The model under review builds one solid part; all positions refer to its coordinate system, in mm. Face numbers are marked on the shaded views. A direction names the side the tool comes from. Coordinates: 2 decimals unless noted, no trailing zeros. Order: outer loops, then holes, each group sorted by start corner. A loop starts at its lowest first (then second) coordinate and runs counter-clockwise, first axis right, second up. Notation, with made-up numbers: (39.5, 61) -> (86.5, 61) arc R28 cw to (86.5, 88) -> close; hole circle Ø8 at (54, 4). An arc over 180 degrees is marked (long way). Use one line per item in the form item = value.
from build123d import *

# Parameters (mm, degrees)
SKETCH1_R           = 12.7
BOSS_EXTRUDE1_DEPTH = 5
SKETCH1_3_R         = 6
CUT_EXTRUDE1_DEPTH  = 5
SKETCH1_4_R         = 7.5
SKETCH1_4_R_2       = 6
CUT_EXTRUDE2_DEPTH  = 2.5
CHAMFER1_SIZE       = 0.25


with BuildPart() as part:
    # Sketch1 → Boss-Extrude1 (new body)
    with BuildSketch(Plane(origin=(0, 0, 0), x_dir=(1, 0, 0), z_dir=(0, 1, 0))):
        with Locations(Location((0, 0, 0), (0, 0, 270))):
            Circle(SKETCH1_R)
    extrude(amount=BOSS_EXTRUDE1_DEPTH)

    # Sketch1<3> → Cut-Extrude1 (cut)
    with BuildSketch(Plane(origin=(0, 0, 0), x_dir=(1, 0, 0), z_dir=(0, 1, 0))):
        with Locations(Location((0, 0, 0), (0, 0, 270))):
            Circle(SKETCH1_3_R)
    extrude(amount=CUT_EXTRUDE1_DEPTH, mode=Mode.SUBTRACT)

    # Sketch1<4> → Cut-Extrude2 (cut)
    with BuildSketch(Plane(origin=(0, 0, 0), x_dir=(1, 0, 0), z_dir=(0, 1, 0))):
        with Locations(Location((0, 0, 0), (0, 0, 270))):
            Circle(SKETCH1_4_R)
        with Locations(Location((0, 0, 0), (0, 0, 270))):
            Circle(SKETCH1_4_R_2, mode=Mode.SUBTRACT)
    extrude(amount=CUT_EXTRUDE2_DEPTH, mode=Mode.SUBTRACT)

    # Chamfer1
    chamfer1_edges = [part.edges().sort_by_distance(p)[0] for p in [
        (0, 0, -7.5),
        (0, 0, -12.7),
        (0, 5, -12.7),
    ]]
    chamfer(chamfer1_edges, length=CHAMFER1_SIZE)


solid = part.part
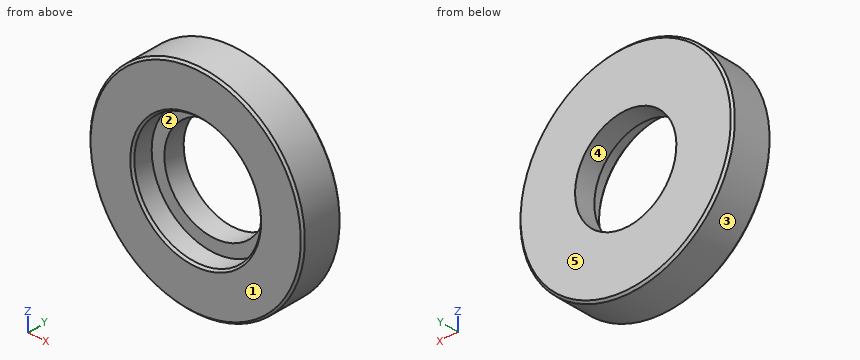
Item 1: We need section C-C (y = 4.35). Write out the cut boundary in (x, z), plus the area to 3 significant figures.
Results found:
outline = circle Ø25.4 at (0, 0); hole circle Ø12 at (0, 0)
area = 394 mm²
Item 2: To check wall thickness, follow L1, parallel to X at y = 1.35, z = 0; L2, parallel to X at y = 4.25, z = 0; L3, parallel to Y at x = -3.5, z = -6.5. State the ranges of each line that lie inside material, in increasing order. Write a range as from..to.
Results found:
L1 = -12.7..-7.5, 7.5..12.7
L2 = -12.7..-6, 6..12.7
L3 = 2.5..5
Item 3: Tool access review of the marked faces 1 and 2: name each direction out of +Z, -Z, +X, -X, +Y, -Y from which nothing blocks a thin tool from reaching the whole face with its end or side.
Results found:
face_1 = +Z, -Z, +X, -X, -Y
face_2 = -Y
Item 4: We need section B-B (x = 0). Write out the cut boundary in (y, z), plus the area to 3 significant figures.
Results found:
outline = (0, -12.45) -> (0.25, -12.7) -> (4.75, -12.7) -> (5, -12.45) -> (5, -6) -> (2.5, -6) -> (2.5, -7.5) -> (0.25, -7.5) -> (0, -7.75) -> close; (0, 7.75) -> (0.25, 7.5) -> (2.5, 7.5) -> (2.5, 6) -> (5, 6) -> (5, 12.45) -> (4.75, 12.7) -> (0.25, 12.7) -> (0, 12.45) -> close
area = 59.3 mm²
Item 5: We need section A-A (z = 0). Write out the cut boundary in (x, y).
Results found:
outline = (-12.7, 0.25) -> (-12.45, 0) -> (-7.75, 0) -> (-7.5, 0.25) -> (-7.5, 2.5) -> (-6, 2.5) -> (-6, 5) -> (-12.45, 5) -> (-12.7, 4.75) -> close; (6, 2.5) -> (7.5, 2.5) -> (7.5, 0.25) -> (7.75, 0) -> (12.45, 0) -> (12.7, 0.25) -> (12.7, 4.75) -> (12.45, 5) -> (6, 5) -> close
Item 6: Clearance check with a flat-ended pin moving along its axis: pin 1 (13.5 mm diameter, centred on x = 0, z = 0, fed in from -Y). State where the tip first meets the part, or that it passes through.
Results found:
pin_1 = 2.5
Item 7: Draft analysis for pull direction X (two halves, no side actions). For the marked faces 3, 4 and 5, state which applies: released by +X, released by -X, zero draft, split by the parting line, or undercut.
Results found:
face_3 = split by the parting line
face_4 = undercut
face_5 = zero draft
